Verification items for the finished model (mm, model axes). A direction names the side the tool comes from. Give positions to 0.01 mm unless a question says otherwise; leave off trailing zeros. Loops run counter-clockwise (first coordinate to the right, second up) from the corner with the lowest first, then second, coordinate; pieces in that order, holes last. Notation, with made-up numbers: M -34,63 L -4,63 A15 ccw -4,67 Z; hole C 89,75 d8. An arc over 180 degrees is marked long. Put each result on its own line as item: value. Start each with the question number.
from build123d import *

# Parameters (mm, degrees)
SKETCH1_R           = 152.4
SKETCH1_R_2         = 146.05
BOSS_EXTRUDE1_DEPTH = 438.15
SKETCH2_W           = 70.919063033
SKETCH2_H           = 12.7
CUT_EXTRUDE1_DEPTH  = 400.05
SKETCH3_W           = 12.7
SKETCH3_H           = 25.42329985
CUT_EXTRUDE2_DEPTH  = 508


with BuildPart() as part:
    # Sketch1 → Boss-Extrude1 (new body)
    with BuildSketch(Plane.XY):
        Circle(SKETCH1_R)
        Circle(SKETCH1_R_2, mode=Mode.SUBTRACT)
    extrude(amount=BOSS_EXTRUDE1_DEPTH)

    # Sketch2 → Cut-Extrude1 (cut, symmetric)
    with BuildSketch(Plane(origin=(0, 0, 0), x_dir=(1, 0, 0), z_dir=(0, 1, 0))):
        with Locations((-0.319607005, -228.6)):
            Rectangle(SKETCH2_W, SKETCH2_H)
    extrude(amount=CUT_EXTRUDE1_DEPTH, both=True, mode=Mode.SUBTRACT)

    # Sketch3 → Cut-Extrude2 (cut)
    with BuildSketch(Plane(origin=(0, 0, 0), x_dir=(0, 0, -1), z_dir=(1, 0, 0))):
        with Locations((-228.6, 0)):
            Rectangle(SKETCH3_W, SKETCH3_H)
    extrude(amount=-CUT_EXTRUDE2_DEPTH, mode=Mode.SUBTRACT)


solid = part.part
Q1. Cross-section at A-A, the plane y = 0. Record the boundary of the cut face in (x, z), then the cut area to 3 significant figures.
Q2. Cross-section at C-C, the plane y = 68.5. Record the boundary of the cut face in (x, z), then the cut area to 3 significant figures.
Q3. Set-up check for faces 1 (the face through (-1, 148, 234.95)), 2 (the face through (139.306, 43.869, 216.008)): record each of +Z, -Z, +X, -X, +Y, -Y from which the full face is reachable in a straight line by a thin tool's end or side.
Q4. Cross-section at B-B, the plane x = 0. Record the boundary of the cut face in (y, z), then the cut area to 3 significant figures.
Q5. Scan lines: L1, parallel to Y at x = 3, z = 69; L2, parallel to X at y = 4.5, z = 368; L3, parallel to X at y = 51.5, z = 248.5. Record each from-to range of solid material in increasing order.
Q6. Release check for a two-part mould opening along X. For faces 3 (the face through (-120.94, -92.73, 216.01)), 4 (the face through (-1, -148, 234.95)), 5 (the face through (78.3, -123.5, 438.15)), 6 (the face through (-1, -148, 222.25)) record: pulls with the +X half, pulls with the -X half, needs draft (parallel to the pull), parting line crosses it, or undercut.
Q7. Go/stop test with flat-tipped pins: pin 1 (1 mm diameter, centred on y = -22, z = 186.5, fed in from +X); pin 2 (8.5 mm diameter, centred on x = -0.5, y = 144.5, fed in from +Z); pin 3 (6 mm diameter, centred on y = -45.5, z = 250.5, fed in from -X); pin 4 (6 mm diameter, centred on x = 103.5, z = 120, fed in from +Y). Record where each tip stops, or that it passes through.
Q8. Cross-section at D-D, the plane x = 52.5. Record the boundary of the cut face in (y, z).
Ans:
1. outline: M -152.4,0 L -146.05,0 L -146.05,222.25 L -152.4,222.25 Z; M -152.4,234.95 L -146.05,234.95 L -146.05,438.15 L -152.4,438.15 Z; M 146.05,0 L 152.4,0 L 152.4,438.15 L 146.05,438.15 Z
1. area: 5,480 mm^2
2. outline: M -136.14,0 L -128.99,0 L -128.99,438.15 L -136.14,438.15 Z; M 128.99,0 L 136.14,0 L 136.14,438.15 L 128.99,438.15 Z
2. area: 6,260 mm^2
3. face 1: +Y, -Y
3. face 2: +Z, -Z
4. outline: M -152.4,0 L -146.05,0 L -146.05,222.25 L -152.4,222.25 Z; M -152.4,234.95 L -146.05,234.95 L -146.05,438.15 L -152.4,438.15 Z; M 146.05,0 L 152.4,0 L 152.4,222.25 L 146.05,222.25 Z; M 146.05,234.95 L 152.4,234.95 L 152.4,438.15 L 146.05,438.15 Z
4. area: 5,400 mm^2
5. L1: y = -152.37 to -146.02, 146.02 to 152.37
5. L2: x = -152.33 to -145.98, 145.98 to 152.33
5. L3: x = -143.43 to -136.67, 136.67 to 143.43
6. face 3: parting line crosses it
6. face 4: undercut
6. face 5: needs draft
6. face 6: undercut
7. pin 1: stops at x = 150.88
7. pin 2: stops at z = 438.15
7. pin 3: stops at x = -146.35
7. pin 4: stops at y = 114.57
8. outline: M -143.07,0 L -136.29,0 L -136.29,438.15 L -143.07,438.15 Z; M 136.29,0 L 143.07,0 L 143.07,438.15 L 136.29,438.15 Z
